from build123d import *

# Parameters (mm, degrees)
F0_R     = 12.7
F1_DEPTH = 1879.6
F2_SIZE2 = 2.032
F2_SIZE  = 2.032
F3_SIZE2 = 2.032
F3_SIZE  = 2.032


with BuildPart() as f1:
    # F0 (on Front) → F1 (new body)
    with BuildSketch(Plane.XZ):
        Circle(F0_R)
    extrude(amount=F1_DEPTH)

    # F2
    f2_edges = [f1.edges().sort_by_distance(p)[0] for p in [
        (-12.7, -1879.6, 0),
    ]]
    chamfer(f2_edges, length=F2_SIZE, length2=F2_SIZE2)

    # F3
    f3_edges = [f1.edges().sort_by_distance(p)[0] for p in [
        (-12.7, 0, 0),
    ]]
    chamfer(f3_edges, length=F3_SIZE, length2=F3_SIZE2)


solid = f1.part
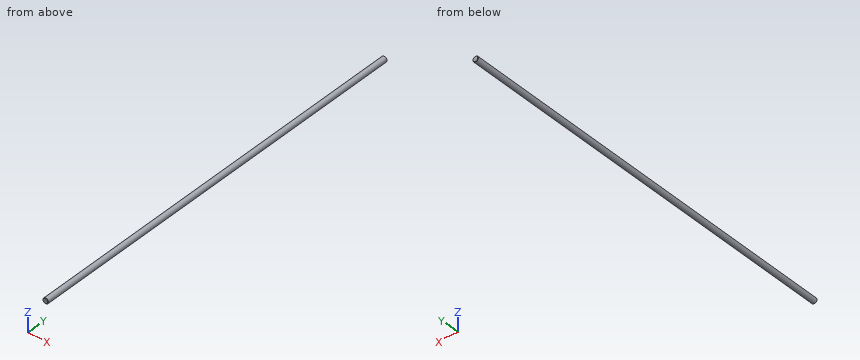
Geometry: final body of the model. Coordinates: model frame, mm. Give positions to 0.01 mm unless a question says otherwise; leave off trailing zeros. Order: outer loops, then holes, each group sorted by start corner. A loop starts at its lowest first (then second) coordinate and runs counter-clockwise, first axis right, second up. Notation, with made-up numbers: (77, -27) -> (109, -27) arc R31 ccw to (109, -1) -> close; hole circle Ø1 at (82, -26.5). An arc over 180 degrees is marked (long way). Answer as a JSON object with one key per item and string values.
Q1. Material intervals for probe 1 along X at (y, z) = (-572.5, -1); probe 2 along Z at (x, y) = (2.25, -1488); probe 3 along X at (y, z) = (-918.5, -1.5), sorted ascending.
Entries:
{"probe 1": "x = -12.66 to 12.66", "probe 2": "z = -12.5 to 12.5", "probe 3": "x = -12.61 to 12.61"}
Q2. Section A-A (y = -1334.5). Output: boundary loops of the cut face in (x, z), plus the area to 3 significant figures.
Entries:
{"outline": "circle Ø25.4 at (0, 0)", "area": "507 mm^2"}
Q3. First-contact query: pin 1 (3 mm diameter, centred on y = -748.5, z = -1.5, fed in from -X); pin 2 (5 mm diameter, centred on y = -911.5, z = -7.5, fed in from +X); pin 3 (2 mm diameter, centred on x = -3.5, y = -224.5, fed in from +Z); pin 4 (1 mm diameter, centred on x = 8, z = 9, fed in from -Y). Flat tips, straight axial feed; report the tip coordinate or a pass-through.
Entries:
{"pin 1": "stops at x = -12.7", "pin 2": "stops at x = 11.67", "pin 3": "stops at z = 12.45", "pin 4": "stops at y = -1878.73"}
